Read the model definition and answer for the solid it produces. Units are mm, in the model's axes. Face numbers are marked on the shaded views. A direction names the side the tool comes from. Give positions to 0.01 mm unless a question says otherwise; leave off trailing zeros. Loops run counter-clockwise (first coordinate to the right, second up) from the corner with the lowest first, then second, coordinate; pieces in that order, holes last. Notation, with made-up numbers: (50.25, 29) - (82.25, 29) arc R25 cw to (82.25, 54) - close; hole circle Ø6 at (8.5, 79). An arc over 180 degrees is marked (long way). Write item = value, one per line.
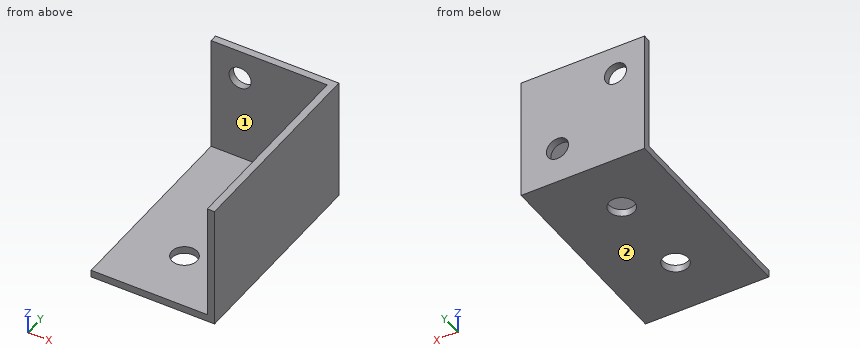
Autodesk Inventor part; units mm, degrees
ref_plane "YZ Plane" through (0, 0, 0) normal (1, 0, 0) x (0, 1, 0)
ref_plane "XZ Plane" through (0, 0, 0) normal (0, 1, 0) x (-1, 0, 0)
ref_plane "XY Plane" through (0, 0, 0) normal (0, 0, 1) x (1, 0, 0)
sketch "Sketch1" plane through (0, 0, 0) normal (0, 1, 0) x (-1, 0, 0)
  line L0 (0, 0) -> (25.4, 0)
  line L1 (25.4, 0) -> (25.4, -25.4)
  line L2 (25.4, -25.4) -> (0, -25.4)
  line L3 (0, -25.4) -> (0, 0)
  line L4 (-1.5875, 1.5875) -> (26.9875, 1.5875)
  line L5 (26.9875, 1.5875) -> (26.9875, -26.9875)
  line L6 (26.9875, -26.9875) -> (-1.5875, -26.9875)
  line L7 (-1.5875, -26.9875) -> (-1.5875, 1.5875)
  circle A0 centre (19.05, -6.35) radius 2.413
  line L8 (0, 0) -> (25.4, -25.4) construction
  circle A1 centre (6.35, -19.05) radius 2.413
  dimension "d0" = 25.4
  dimension "d1" = 25.4
  dimension "d2" = 1.5875
  dimension "d3" = 4.826
  dimension "d4" = 6.35
  dimension "d5" = 6.35
extrude "Extrusion1" add sketch "Sketch1" against normal blind 1.5875 contours L0 L1 L2 L3 | L4 L5 L6 L7
extrude "Extrusion2" add sketch "Sketch1" against normal blind 44.7675 contours L4 L5 L6 L7
sketch "Sketch2" plane through (1.5875, 0, -26.9875) normal (0, 0, -1) x (-1, 0, 0)
  line L0 (0, 0) -> (28.575, 0) construction
  line L1 (14.2875, 0) -> (14.2875, -44.7675) construction
  line L2 (1.5875, -44.7675) -> (26.9875, -44.7675) construction
  circle A0 centre (14.2875, -12.7) radius 2.7781
  circle A1 centre (14.2875, -32.0675) radius 2.7781
  point P0 (1.5875, 0)
  dimension "d10" = 5.5563
  dimension "d11" = 12.7
  dimension "d12" = 12.7
extrude "Extrusion3" cut sketch "Sketch2" against normal blind 44.7675
sketch "Sketch3" plane through (-26.9875, 0, -26.9875) normal (-1, 0, 0) x (0, 0, 1)
  line L0 (0, 0) -> (28.575, 0)
  line L1 (0, 0) -> (0, -44.7675)
  line L2 (28.575, -44.7675) -> (0, -44.7675)
  line L3 (28.575, 0) -> (28.575, -44.7675)
  point P0 (26.9875, 0)
sketch "Sketch4" plane through (-26.9875, 0, 1.5875) normal (0, 0, 1) x (1, 0, 0)
  circle A0 centre (14.2875, -32.0675) radius 2.7781
  circle A1 centre (14.2875, -12.7) radius 2.7781
  line L0 (0, 0) -> (28.575, 0)
  line L1 (0, 0) -> (0, -44.7675)
  line L2 (28.575, -44.7675) -> (0, -44.7675)
  line L3 (28.575, 0) -> (28.575, -44.7675)
  point P0 (26.9875, 0)
extrude "Extrusion4" cut sketch "Sketch3" against normal blind 1.5875
extrude "Extrusion5" cut sketch "Sketch4" against normal blind 1.5875
properties part number "FlipperTensionerBlock1Tool"
1) Each of these flat-tipped pins is pushed along its axis until it touches: P1, Ø12.5, axis at y = -24.5, z = -16, coming from the -X side; P2, Ø9, axis at x = -12.7, y = -12.7, coming from the +Z side; P3, Ø5, axis at x = -12.7, y = -32.07, coming from the -Z side; P4, Ø12.5, axis at x = -13, z = -11, coming from the -Y side. Where does it stop, or does it pass through?
Output:
P1 = 0
P2 = -25.4
P3 = through
P4 = -1.59
2) A cutting plane is placed at C-C on x = -12.7. Determine the outline of the cut face in (y, z), then the cut area to 4 significant figures.
Output:
outline = (-44.77, -26.99) - (-34.85, -26.99) - (-34.85, -25.4) - (-44.77, -25.4) - close; (-29.29, -26.99) - (-15.48, -26.99) - (-15.48, -25.4) - (-29.29, -25.4) - close; (-9.92, -26.99) - (0, -26.99) - (0, 0) - (-1.59, 0) - (-1.59, -25.4) - (-9.92, -25.4) - close
area = 93.75 mm²
3) Find the intervals of material crossed by probe 1 along Y at (x, z) = (-12.7, -26.5); probe 2 along Z at (x, y) = (-2.75, -12); probe 3 along X at (y, z) = (-40, -8.75), in increasing order.
Output:
probe_1 = -44.77 to -34.85, -29.29 to -15.48, -9.92 to 0
probe_2 = -26.99 to -25.4
probe_3 = 0 to 1.59
4) A cutting plane is placed at B-B on y = -12.7. Determine the outline of the cut face in (x, z).
Output:
outline = (-25.4, -26.99) - (-15.48, -26.99) - (-15.48, -25.4) - (-25.4, -25.4) - close; (-9.92, -26.99) - (1.59, -26.99) - (1.59, 0) - (0, 0) - (0, -25.4) - (-9.92, -25.4) - close
5) A tool of negligible diameter and unlimited length cuts with its end or side. For the marked faces 1 and 2, from which of +Z, -Z, +X, -X, +Y, -Y can it reach the whole face along a straight path? Write none if from no direction.
Output:
face_1 = +Z, -X, -Y
face_2 = -Z, +X, -X, +Y, -Y
6) A cutting plane is placed at A-A on x = -6.35. Determine the outline of the cut face in (y, z), then the cut area to 3 significant figures.
Output:
outline = (-44.77, -26.99) - (0, -26.99) - (0, -21.46) - (-1.59, -21.46) - (-1.59, -25.4) - (-44.77, -25.4) - close; (-1.59, -16.64) - (0, -16.64) - (0, 0) - (-1.59, 0) - close
area = 104 mm²
7) A cutting plane is placed at D-D on y = -19.5. Determine the outline of the cut face in (x, z), then the cut area to 3 significant figures.
Output:
outline = (-25.4, -26.99) - (1.59, -26.99) - (1.59, 0) - (0, 0) - (0, -25.4) - (-25.4, -25.4) - close
area = 83.2 mm²
